```python
from build123d import *

# Parameters (mm, degrees)
BOSS_EXTRUDE1_DEPTH = 13
BOSS_EXTRUDE2_DEPTH = 3


with BuildPart() as part:
    # Sketch2 → Boss-Extrude1 (new body)
    with BuildSketch(Plane(origin=(0, 0, 0), x_dir=(1, 0, 0), z_dir=(0, 1, 0))):
        with BuildLine():
            Line((-71.350602173, 25), (-61.081912216, 25))
            ThreePointArc((-61.081912216, 25), (0, 66), (61.081912216, 25))
            Line((61.081912216, 25), (71.350602173, 25))
            Line((71.350602173, 25), (71.350602173, 30))
            Line((71.350602173, 30), (64.350602173, 30))
            ThreePointArc((64.350602173, 30), (0, 71), (-64.350602173, 30))
            Line((-64.350602173, 30), (-71.350602173, 30))
            Line((-71.350602173, 30), (-71.350602173, 25))
        make_face()
    extrude(amount=BOSS_EXTRUDE1_DEPTH)

    # Sketch3 → Boss-Extrude2 (add)
    with BuildSketch(Plane.XZ):
        with BuildLine():
            Line((66.452990903, -25), (61.081912216, -25))
            ThreePointArc((61.081912216, -25), (0, -66), (-61.081912216, -25))
            Line((-61.081912216, -25), (-66.452990903, -25))
            ThreePointArc((-66.452990903, -25), (0, -71), (66.452990903, -25))
        make_face()
    extrude(amount=BOSS_EXTRUDE2_DEPTH)


solid = part.part
```
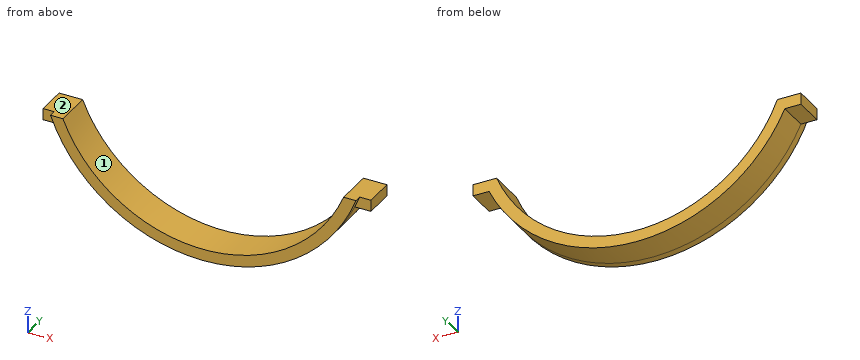
Read the model definition and answer for the solid it produces. Units are mm, in the model's axes. Face numbers are marked on the shaded views. Give positions to 0.01 mm unless a question says otherwise; leave off trailing zeros. Write each loop counter-clockwise with the first axis right and the second up, starting at its lowest first coordinate (ties: lowest second). Pieces come first, ordered by that corner, then holes. Notation, with made-up numbers: (49, 6) -> (101, 6) arc R7 cw to (101, 10) -> close; hole circle Ø3 at (-23, -19). An arc over 180 degrees is marked (long way). Answer in a Markdown table with one row per item.
1) Section D-D on z = -35.5 is taken. Give the vertices of the cut face in (x, y), plus the area to 3 significant figures.
Results list:
| item | result |
|---|---|
| outline | (-61.49, -3) -> (-55.64, -3) -> (-55.64, 13) -> (-61.49, 13) -> close; (55.64, -3) -> (61.49, -3) -> (61.49, 13) -> (55.64, 13) -> close |
| area | 187 mm^2 |
2) Determine the mould class of the marked faces 1 and 2 for opening direction X: released by +X, released by -X, zero draft, split by the parting line, or undercut.
Results list:
| item | result |
|---|---|
| face 1 | undercut |
| face 2 | zero draft |
3) Section C-C on x = 25 is taken. Give the vertices of the cut face in (y, z).
Results list:
| item | result |
|---|---|
| outline | (-3, -66.45) -> (13, -66.45) -> (13, -61.08) -> (-3, -61.08) -> close |
4) Section B-B on y = 9.5 is taken. Give the vertices of the cut face in (x, z).
Results list:
| item | result |
|---|---|
| outline | (-71.35, -30) -> (-64.35, -30) arc R71 ccw to (64.35, -30) -> (71.35, -30) -> (71.35, -25) -> (61.08, -25) arc R66 cw to (-61.08, -25) -> (-71.35, -25) -> close |
5) Section A-A on z = -63 is taken. Give the vertices of the cut face in (x, y), plus the area to 3 significant figures.
Results list:
| item | result |
|---|---|
| outline | (-32.74, -3) -> (-19.67, -3) -> (-19.67, 13) -> (-32.74, 13) -> close; (19.67, -3) -> (32.74, -3) -> (32.74, 13) -> (19.67, 13) -> close |
| area | 418 mm^2 |
6) Straight lines are drawn through the part: line 1 (X direction, y = 11.25, z = -39); line 2 (Z direction, x = -1.5, y = 6.75); line 3 (X direction, y = 0.25, z = -57.5). For each, find the intervals that lie inside material, in ascending order. Write a range as [from, to].
Results list:
| item | result |
|---|---|
| line 1 | [-59.33, -53.24], [53.24, 59.33] |
| line 2 | [-70.98, -65.98] |
| line 3 | [-41.65, -32.4], [32.4, 41.65] |
7) Each of these flat-tipped pins is pushed along its axis until it touches: pin 1 Ø6 at (x, y) = (8, 1.5) entering from +Z; pin 2 Ø1 at (y, z) = (4, -61) entering from -X; pin 3 Ø2.5 at (x, z) = (-67.5, -28) entering from -Y. Where does it stop, or does it pass through?
Results list:
| item | result |
|---|---|
| pin 1 | z = -65.08 |
| pin 2 | x = -37.16 |
| pin 3 | y = 0 |
